```python
from build123d import *

# Parameters (mm, degrees)
SKETCH1_W           = 45.212
SKETCH1_H           = 1.27
BOSS_EXTRUDE2_DEPTH = 2.54
SKETCH1_5_W         = 45.212
SKETCH1_5_H         = 3.81
BOSS_EXTRUDE3_DEPTH = 1.778
BOSS_EXTRUDE4_START = 1.524
BOSS_EXTRUDE4_DEPTH = 1.27
BOSS_EXTRUDE5_DEPTH = 14.986
SKETCH2_W           = 0.508
SKETCH2_H           = 8.128
CUT_EXTRUDE1_DEPTH  = 76.866530328


with BuildPart() as part:
    # Sketch1 → Boss-Extrude2 (new body)
    with BuildSketch(Plane(origin=(0, 0, 0), x_dir=(0, 0, -1), z_dir=(1, 0, 0))):
        with BuildLine():
            ThreePointArc((4.318, 0), (3.053287081, 3.053287081), (0, 4.318))
            Line((0, 4.318), (0, -4.318))
            ThreePointArc((0, -4.318), (3.053287081, -3.053287081), (4.318, 0))
        make_face()
        with BuildLine():
            Line((0, -4.318), (0, 4.318))
            ThreePointArc((0, 4.318), (-4.318, 0), (0, -4.318))
        make_face()
        with BuildLine():
            ThreePointArc((0, -4.318), (-4.318, 0), (0, 4.318))
            Line((0, 4.318), (-9.398, 4.318))
            Line((-9.398, 4.318), (-9.398, 1.244340789))
            ThreePointArc((-9.398, 1.244340789), (-8.340781474, 0.98373777), (-7.874, 0))
            ThreePointArc((-7.874, 0), (-8.340781474, -0.98373777), (-9.398, -1.244340789))
            Line((-9.398, -1.244340789), (-9.398, -4.318))
            Line((-9.398, -4.318), (0, -4.318))
        make_face()
        with BuildLine():
            Line((-9.398, 1.244340789), (-9.398, 4.318))
            ThreePointArc((-9.398, 4.318), (-11.932525974, 3.495897895), (-13.501957395, 1.342630889))
            ThreePointArc((-13.501957395, 1.342630889), (-15.817903355, -1.834857441), (-19.558, -3.048))
            Line((-19.558, -3.048), (-19.558, -4.318))
            Line((-19.558, -4.318), (-9.398, -4.318))
            Line((-9.398, -4.318), (-9.398, -1.244340789))
            ThreePointArc((-9.398, -1.244340789), (-10.414, 0), (-9.398, 1.244340789))
        make_face()
        with Locations((-42.164, -3.683)):
            Rectangle(SKETCH1_W, SKETCH1_H)
        Polygon((-69.679321023, -4.318), (-64.77, -4.318), (-64.77, -3.048), (-70.05358602, -3.048), align=None)
        with BuildLine():
            ThreePointArc((-7.874, 0), (-8.340781474, 0.98373777), (-9.398, 1.244340789))
            Line((-9.398, 1.244340789), (-9.398, -1.244340789))
            ThreePointArc((-9.398, -1.244340789), (-8.340781474, -0.98373777), (-7.874, 0))
        make_face()
        with BuildLine():
            Line((-9.398, -1.244340789), (-9.398, 1.244340789))
            ThreePointArc((-9.398, 1.244340789), (-10.414, 0), (-9.398, -1.244340789))
        make_face()
    extrude(amount=BOSS_EXTRUDE2_DEPTH)

    # Sketch1_5 → Boss-Extrude3 (add)
    with BuildSketch(Plane(origin=(0, 0, 0), x_dir=(0, 0, -1), z_dir=(1, 0, 0))):
        Polygon((-19.558, -8.128), (-9.398, -4.318), (-19.558, -4.318), align=None)
        with Locations((-42.164, -6.223)):
            Rectangle(SKETCH1_5_W, SKETCH1_5_H)
        Polygon((-68.55652603, -8.128), (-64.77, -8.128), (-64.77, -4.318), (-69.679321023, -4.318), align=None)
    extrude(amount=BOSS_EXTRUDE3_DEPTH)

    # Sketch1_7 → Boss-Extrude4 (add)
    with BuildSketch(Plane(origin=(0, 0, 0), x_dir=(0, 0, -1), z_dir=(1, 0, 0)).offset(BOSS_EXTRUDE4_START)):
        Polygon((-70.05358602, -3.048), (-64.77, -3.048), (-64.77, 0.508), (-67.200502007, 0.508), (-67.200502007, 4.064), (-64.77, 4.064), (-64.77, 6.604), (-72.898, 6.604), align=None)
    extrude(amount=-BOSS_EXTRUDE4_DEPTH)

    # Sketch1_8 → Boss-Extrude5 (add)
    with BuildSketch(Plane(origin=(0, 0, 0), x_dir=(0, 0, -1), z_dir=(1, 0, 0))):
        with BuildLine():
            ThreePointArc((-7.874, 0), (-8.340781474, 0.98373777), (-9.398, 1.244340789))
            Line((-9.398, 1.244340789), (-9.398, -1.244340789))
            ThreePointArc((-9.398, -1.244340789), (-8.340781474, -0.98373777), (-7.874, 0))
        make_face()
        with BuildLine():
            Line((-9.398, -1.244340789), (-9.398, 1.244340789))
            ThreePointArc((-9.398, 1.244340789), (-10.414, 0), (-9.398, -1.244340789))
        make_face()
    extrude(amount=-BOSS_EXTRUDE5_DEPTH)

    # Sketch2 → Cut-Extrude1 (cut, through all)
    with BuildSketch(Plane(origin=(0, 6.604, 0), x_dir=(1, 0, 0), z_dir=(0, 1, 0))):
        with Locations((0.254, -68.834)):
            Rectangle(SKETCH2_W, SKETCH2_H)
    extrude(amount=-CUT_EXTRUDE1_DEPTH, mode=Mode.SUBTRACT)


solid = part.part
```
Can you work these out from the model? Positions are in its coordinate system, mm. A direction names the side the tool comes from. Coordinates: 2 decimals unless noted, no trailing zeros. Loops run counter-clockwise (first coordinate to the right, second up) from the corner with the lowest first, then second, coordinate; pieces in that order, holes last. Notation, with made-up numbers: (-12, 87.25) - (21, 87.25) arc R19 ccw to (21, 120.25) - close; hole circle Ø7 at (16.25, 66). An arc over 180 degrees is marked (long way). Use a Markdown table: item, result.
Item 1: For faces 5 (the face through (1.25, -1.8, 15.77)), 6 (the face through (2, -4.318, 28)), 7 (the face through (1, 4.318, 5)), 8 (the face through (0.508, 1, 68)), 9 (the face through (1.524, 2, 69)), which set-ups out of +Z, -Z, +X, -X, +Y, -Y let a thin tool reach every point of the face, with its end or its side?
Numbers:
| item | result |
|---|---|
| face 5 | +X, -X, +Y |
| face 6 | -Z, +X, -Y |
| face 7 | -Z, +X, -X, +Y |
| face 8 | +Z, -X, +Y, -Y |
| face 9 | +Z, +X, +Y |
Item 2: I want a section at C-C on x = -4. Please give me the cut outline in (y, z).
Numbers:
| item | result |
|---|---|
| outline | circle Ø2.54 at (0, 9.14) |
Item 3: We'd pull the mould along Z, two halves only. Please class faces 1 (the face through (1.25, 3.52, 11.9)), 2 (the face through (1, -3.048, 44)), 3 (the face through (1.778, -6, 40)), 4 (the face through (0.88, -6.25, 14.55)): released by +Z, released by -Z, zero draft, split by the parting line, or undercut.
Numbers:
| item | result |
|---|---|
| face 1 | undercut |
| face 2 | undercut |
| face 3 | zero draft |
| face 4 | released by -Z |
Item 4: Will these pins go through, and if not, where does the flat tip stop? pin 1 (3.5 mm diameter, centred on y = -2, z = 29, fed in from -X); pin 2 (0.8 mm diameter, centred on x = 1, y = 2, fed in from -Z); pin 3 (0.5 mm diameter, centred on x = 1, y = -1.5, fed in from -Z).
Numbers:
| item | result |
|---|---|
| pin 1 | stops at x = 0 |
| pin 2 | stops at z = -4.01 |
| pin 3 | stops at z = -4.13 |
Item 5: I want a section at A-A on y = 2.75. Please give me the cut outline in (x, z).
Numbers:
| item | result |
|---|---|
| outline | (0, -3.33) - (2.54, -3.33) - (2.54, 12.73) - (0, 12.73) - close; (0.51, 67.2) - (1.52, 67.2) - (1.52, 71.76) - (0.51, 71.76) - close |
Item 6: I want a section at B-B on z = 40. Please give me the cut outline in (x, y).
Numbers:
| item | result |
|---|---|
| outline | (0, -8.13) - (1.78, -8.13) - (1.78, -4.32) - (2.54, -4.32) - (2.54, -3.05) - (0, -3.05) - close |
Item 7: I want a section at D-D on y = -5. Please give me the cut outline in (x, z).
Numbers:
| item | result |
|---|---|
| outline | (0, 11.22) - (1.78, 11.22) - (1.78, 69.48) - (0.51, 69.48) - (0.51, 64.77) - (0, 64.77) - close |
Item 8: If I drill on probe 1 along X at (y, z) = (-5.5, 21); probe 2 along X at (y, z) = (-2.5, 12.5); probe 3 along Z at (x, y) = (0.75, 4.5), over which ranges is the centre line in solid material (lowest first)? Write a range as from..to.
Numbers:
| item | result |
|---|---|
| probe 1 | x = 0..1.78 |
| probe 2 | x = 0..2.54 |
| probe 3 | z = 64.77..72.28 |
